Check sheet for the modelled part. Datum: model origin and axes. Units: mm. Face numbers are marked on the shaded views. A direction names the side the tool comes from. Round coordinates to 2 decimals unless told otherwise and drop trailing zeros. Write each loop counter-clockwise with the first axis right and the second up, starting at its lowest first coordinate (ties: lowest second). Pieces come first, ordered by that corner, then holes.
Item 1: Section check D-D, the plane z = -0.5. Record the cut outline in (x, y), plus the area to 3 significant figures.
Item 2: Depth check by flat-ended pin: pin 1 (0.6 mm diameter, centred on y = -9, z = 6, fed in from -X) (3 decimals); pin 2 (0.5 mm diameter, centred on x = -5, y = -2.5, fed in from +Z); pin 3 (0.9 mm diameter, centred on x = 6, z = 3.5, fed in from +Y). Enter the tip coordinate at first touch or a pass-through.
Item 3: Section check C-C, the plane z = 6.75. Record the cut outline in (x, y) (3 decimals).
Item 4: Set-up check for the marked faces 4, 5 and 6: record each of +Z, -Z, +X, -X, +Y, -Y from which the full face is reachable in a straight line by a thin tool's end or side.
Item 5: Section check A-A, the plane x = -5. Record the cut outline in (y, z).
Item 6: Release check for a two-part mould opening along Y. For the marked faces 1, 2 and 3 record: pulls with the +Y half, pulls with the -Y half, needs draft (parallel to the pull), parting line crosses it, or undercut.
Item 7: Section check B-B, the plane y = 2.5. Record the cut outline in (x, z), plus the area to 3 significant figures.
Item 8: Material ranges on line 1 along X through (y, z) = (2.5, 8.4); line 2 along Y through (x, z) = (4.75, 3.25); line 3 along Y through (x, z) = (-1.75, -1.25), recorded low to high.
from build123d import *

# Parameters (mm, degrees)
F1_DEPTH = 9.5
F2_R     = 0.5
F3_DEPTH = 2
F4_R     = 2.05
F5_DEPTH = 2.6
F6_R     = 0.2
F8_ANGLE = 90


with BuildPart() as f1:
    # F0 (on Top) → F1 (new body)
    with BuildSketch(Plane.XY):
        Polygon((-9.95, 4.375), (-9.95, 0), (-9.95, -4.375), (-7.9, -4.375), (-7.9, -7.4), (0, -7.4), (7.9, -7.4), (7.9, -4.375), (9.95, -4.375), (9.95, 0), (9.95, 4.375), (7.9, 4.375), (7.9, 7.4), (0, 7.4), (-7.9, 7.4), (-7.9, 4.375), align=None)
    extrude(amount=F1_DEPTH)

    # F2 (on face) → F3 (cut)
    with BuildSketch(Plane.XY.offset(9.5)):
        Circle(F2_R)
        with Locations((0, 2.5)):
            Circle(F2_R)
        with Locations((0, 5)):
            Circle(F2_R)
        with Locations((2.5, 0)):
            Circle(F2_R)
        with Locations((2.5, 2.5)):
            Circle(F2_R)
        with Locations((2.5, 5)):
            Circle(F2_R)
        with Locations((5, 0)):
            Circle(F2_R)
        with Locations((5, 2.5)):
            Circle(F2_R)
        with Locations((5, 5)):
            Circle(F2_R)
        with Locations((-5, 0)):
            Circle(F2_R)
        with Locations((-2.5, 5)):
            Circle(F2_R)
        with Locations((-2.5, 2.5)):
            Circle(F2_R)
        with Locations((-2.5, 0)):
            Circle(F2_R)
        with Locations((-5, 2.5)):
            Circle(F2_R)
        with Locations((-5, 5)):
            Circle(F2_R)
        with Locations((2.5, -5)):
            Circle(F2_R)
        with Locations((2.5, -2.5)):
            Circle(F2_R)
        with Locations((0, -5)):
            Circle(F2_R)
        with Locations((0, -2.5)):
            Circle(F2_R)
        with Locations((-5, -2.5)):
            Circle(F2_R)
        with Locations((5, -2.5)):
            Circle(F2_R)
        with Locations((5, -5)):
            Circle(F2_R)
        with Locations((-2.5, -5)):
            Circle(F2_R)
        with Locations((-5, -5)):
            Circle(F2_R)
        with Locations((-2.5, -2.5)):
            Circle(F2_R)
    extrude(amount=-F3_DEPTH, mode=Mode.SUBTRACT)

    # F4 (on Top) → F5 (join)
    with BuildSketch(Plane.XY):
        with Locations((-4.95, 0)):
            Circle(F4_R)
        with Locations((4.95, 0)):
            Circle(F4_R)
    extrude(amount=-F5_DEPTH)

    # F6
    f6_edges = [f1.edges().sort_by_distance(p)[0] for p in [
        (-7, 0, -2.6),
        (2.9, 0, -2.6),
    ]]
    fillet(f6_edges, radius=F6_R)


with BuildPart() as f1_1:
    # F8: moved
    add(f1.part.rotate(Axis((0, 0, 33.902004), (0, 0, 1)), F8_ANGLE))


solid = f1_1.part
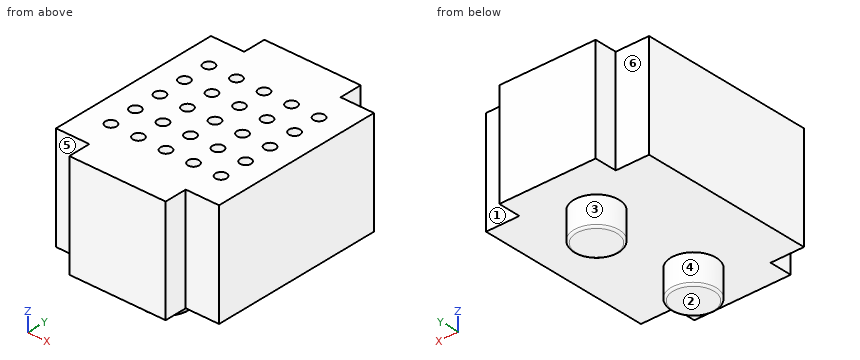
Values found:
1. outline: circle Ø4.1 at (0, -4.95); circle Ø4.1 at (0, 4.95)
1. area: 26.4 mm2
2. pin 1: stops at x = -4.375
2. pin 2: stops at z = 7.5
2. pin 3: stops at y = 7.9
3. outline: (-7.4, -7.9) - (-4.375, -7.9) - (-4.375, -9.95) - (4.375, -9.95) - (4.375, -7.9) - (7.4, -7.9) - (7.4, 7.9) - (4.375, 7.9) - (4.375, 9.95) - (-4.375, 9.95) - (-4.375, 7.9) - (-7.4, 7.9) - close
4. face 4: -Z
4. face 5: +Z, -Z, -X, -Y
4. face 6: +Z, -Z, -X, +Y
5. outline: (-7.9, 0) - (7.9, 0) - (7.9, 9.5) - (5.5, 9.5) - (5.5, 7.5) - (4.5, 7.5) - (4.5, 9.5) - (3, 9.5) - (3, 7.5) - (2, 7.5) - (2, 9.5) - (0.5, 9.5) - (0.5, 7.5) - (-0.5, 7.5) - (-0.5, 9.5) - (-2, 9.5) - (-2, 7.5) - (-3, 7.5) - (-3, 9.5) - (-4.5, 9.5) - (-4.5, 7.5) - (-5.5, 7.5) - (-5.5, 9.5) - (-7.9, 9.5) - close
6. face 1: pulls with the +Y half
6. face 2: needs draft
6. face 3: undercut
7. outline: (-7.4, 0) - (7.4, 0) - (7.4, 9.5) - (5.5, 9.5) - (5.5, 7.5) - (4.5, 7.5) - (4.5, 9.5) - (3, 9.5) - (3, 7.5) - (2, 7.5) - (2, 9.5) - (0.5, 9.5) - (0.5, 7.5) - (-0.5, 7.5) - (-0.5, 9.5) - (-2, 9.5) - (-2, 7.5) - (-3, 7.5) - (-3, 9.5) - (-4.5, 9.5) - (-4.5, 7.5) - (-5.5, 7.5) - (-5.5, 9.5) - (-7.4, 9.5) - close
7. area: 131 mm2
8. line 1: x = -7.4 to -5.5, -4.5 to -3, -2 to -0.5, 0.5 to 2, 3 to 4.5, 5.5 to 7.4
8. line 2: y = -7.9 to 7.9
8. line 3: y = -6.02 to -3.88, 3.88 to 6.02
